Design review of the part built by this model. Coordinates are the model's own, in mm. Coordinates: 2 decimals unless noted, no trailing zeros. Write each loop counter-clockwise with the first axis right and the second up, starting at its lowest first coordinate (ties: lowest second). Pieces come first, ordered by that corner, then holes. Notation, with made-up numbers: M 27,-3 L 84,-3 A18 ccw 84,2 Z; hole C -31.75,81.25 d6. An arc over 180 degrees is marked long. One line per question, with ' | ' between items.
Autodesk Inventor part; units mm, degrees
ref_plane "YZ Plane" through (0, 0, 0) normal (1, 0, 0) x (0, 1, 0)
ref_plane "XZ Plane" through (0, 0, 0) normal (0, 1, 0) x (-1, 0, 0)
ref_plane "XY Plane" through (0, 0, 0) normal (0, 0, 1) x (1, 0, 0)
sketch "草圖1" plane through (0, 0, 0) normal (0, 0, 1) x (1, 0, 0)
  line L0 (31.85, -6) -> (31.85, 6)
  line L1 (-31.85, 6) -> (-31.85, -6)
  line L2 (-30.85, -7) -> (-27.85, -7)
  line L3 (-22.85, -7) -> (22.85, -7)
  line L4 (27.85, -7) -> (30.85, -7)
  line L5 (0, 22.1211) -> (0, -32.4412) construction
  arc A0 (-30.85, 7) -> (-31.85, 6) centre (-30.85, 6) ccw
  arc A1 (-31.85, -6) -> (-30.85, -7) centre (-30.85, -6) ccw
  arc A2 (-27.85, -7) -> (-26.85, -6) centre (-27.85, -6) ccw
  arc A3 (-23.85, -6) -> (-22.85, -7) centre (-22.85, -6) ccw
  arc A4 (30.85, -7) -> (31.85, -6) centre (30.85, -6) ccw
  arc A5 (31.85, 6) -> (30.85, 7) centre (30.85, 6) ccw
  line L6 (-26.85, -6) -> (-26.85, 1)
  line L7 (-26.85, 1) -> (-23.85, 1)
  line L8 (-23.85, 1) -> (-23.85, -6)
  arc A6 (26.85, -6) -> (27.85, -7) centre (27.85, -6) ccw
  arc A7 (22.85, -7) -> (23.85, -6) centre (22.85, -6) ccw
  line L9 (26.85, -6) -> (26.85, 1)
  line L10 (26.85, 1) -> (23.85, 1)
  line L11 (23.85, 1) -> (23.85, -6)
  line L12 (-16.25, 7) -> (-16.25, 1)
  line L13 (-16.25, 1) -> (-13.25, 1)
  line L14 (-13.25, 1) -> (-13.25, 7)
  line L15 (-14.75, -1.2757) -> (-14.75, 3.2757) construction
  line L16 (16.25, 7) -> (16.25, 1)
  line L17 (16.25, 1) -> (13.25, 1)
  line L18 (13.25, 1) -> (13.25, 7)
  line L19 (-31.85, -7) -> (31.85, -7) construction
  line L20 (31.85, -7) -> (31.85, 7) construction
  line L21 (31.85, 7) -> (-31.85, 7) construction
  line L22 (-31.85, 7) -> (-31.85, -7) construction
  line L23 (-31.85, -7) -> (31.85, 7) construction
  line L24 (31.85, -7) -> (-31.85, 7) construction
  line L25 (-16.25, 7) -> (-30.85, 7)
  line L26 (30.85, 7) -> (16.25, 7)
  line L27 (13.25, 7) -> (-13.25, 7)
  line L28 (-26.85, -6) -> (-26.85, -3)
  line L29 (26.85, -3) -> (26.85, -6)
  point P0 (0, 0)
  point P1 (-14.75, 1)
  point P2 (26.85, -6)
  dimension "d5" = 1
  dimension "d6" = 1
  dimension "d25" = 3
  dimension "d26" = 8
  dimension "d28" = 5
  dimension "d29" = 23.85
  dimension "d30" = 6
  dimension "d31" = 3
  dimension "d32" = 14.75
  dimension "d34" = 14
extrude "擠出1" add sketch "草圖1" along normal mid plane 3
properties part number "test"
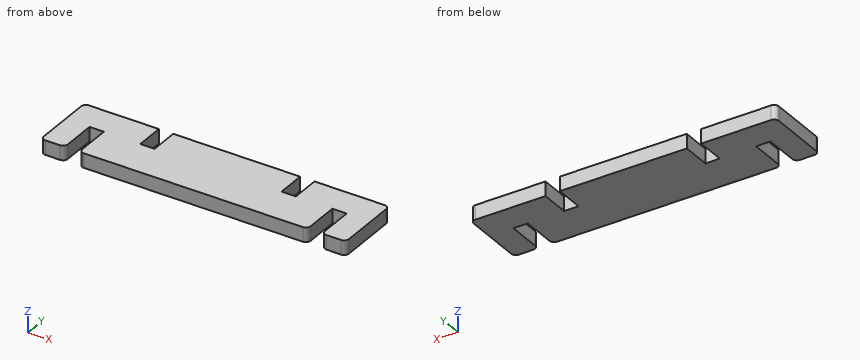
1. Take a section at B-B (z = -0.5). Write out the cut boundary in (x, y).
Answer sheet:
outline: M -31.85,-6 A1 ccw -30.85,-7 L -27.85,-7 A1 ccw -26.85,-6 L -26.85,1 L -23.85,1 L -23.85,-6 A1 ccw -22.85,-7 L 22.85,-7 A1 ccw 23.85,-6 L 23.85,1 L 26.85,1 L 26.85,-6 A1 ccw 27.85,-7 L 30.85,-7 A1 ccw 31.85,-6 L 31.85,6 A1 ccw 30.85,7 L 16.25,7 L 16.25,1 L 13.25,1 L 13.25,7 L -13.25,7 L -13.25,1 L -16.25,1 L -16.25,7 L -30.85,7 A1 ccw -31.85,6 Z
2. Take a section at A-A (y = -5.25). Write out the cut boundary in (x, z), then the cut area to 3 significant figures.
Answer sheet:
outline: M -31.85,-1.5 L -26.85,-1.5 L -26.85,1.5 L -31.85,1.5 Z; M -23.85,-1.5 L 23.85,-1.5 L 23.85,1.5 L -23.85,1.5 Z; M 26.85,-1.5 L 31.85,-1.5 L 31.85,1.5 L 26.85,1.5 Z | area: 173 mm^2
3. Insertion check: pin 1 Ø1.5 at (x, z) = (15, -0.5) entering from +Y; pin 2 Ø1.5 at (x, z) = (25, 0) entering from -Y. Each pin has a flat end and moves straight along its axis. Give the tip position at first contact, or say it passes through.
Answer sheet:
pin 1: y = 1 | pin 2: y = 1
4. To check wall thickness, follow line 1 along X through (y, z) = (4.5, 0.75); line 2 along X through (y, z) = (-5.25, 0.9); line 3 along Y through (x, z) = (24, 0.5). State the ranges of each line that lie inside material, in increasing order. Write a range as [from, to].
Answer sheet:
line 1: [-31.85, -16.25], [-13.25, 13.25], [16.25, 31.85] | line 2: [-31.85, -26.85], [-23.85, 23.85], [26.85, 31.85] | line 3: [1, 7]
5. Take a section at C-C (x = 25). Write out the cut boundary in (y, z), then the cut area to 3 significant figures.
Answer sheet:
outline: M 1,-1.5 L 7,-1.5 L 7,1.5 L 1,1.5 Z | area: 18.0 mm^2
6. Take a section at D-D (x = 14.5). Write out the cut boundary in (y, z).
Answer sheet:
outline: M -7,-1.5 L 1,-1.5 L 1,1.5 L -7,1.5 Z
